```python
from build123d import *

# Parameters (mm, degrees)
SKETCH1_R           = 4.25
BOSS_EXTRUDE1_DEPTH = 55.3238373
CUT_EXTRUDE1_DEPTH  = 6.6
CHAMFER1_SIZE       = 0.5
CUT_EXTRUDE2_DEPTH  = 6.6
CHAMFER2_SIZE       = 0.5


with BuildPart() as part:
    # Sketch1 → Boss-Extrude1 (new body)
    with BuildSketch(Plane(origin=(0, 0, 0), x_dir=(1, 0, 0), z_dir=(0, 1, 0))):
        Circle(SKETCH1_R)
    extrude(amount=BOSS_EXTRUDE1_DEPTH)

    # Sketch2 → Cut-Extrude1 (cut)
    with BuildSketch(Plane(origin=(0, 55.3238373, 0), x_dir=(1, 0, 0), z_dir=(0, 1, 0))):
        Polygon((1.610807251, 2.79), (-1.610807251, 2.79), (-3.221614502, 0), (-1.610807251, -2.79), (1.610807251, -2.79), (3.221614502, 0), align=None)
    extrude(amount=-CUT_EXTRUDE1_DEPTH, mode=Mode.SUBTRACT)

    # Chamfer1
    chamfer1_edges = [part.edges().sort_by_distance(p)[0] for p in [
        (2.416210877, 55.3238373, -1.395),
        (0, 55.3238373, -2.79),
        (-2.416210877, 55.3238373, -1.395),
        (-2.416210877, 55.3238373, 1.395),
        (0, 55.3238373, 2.79),
        (2.416210877, 55.3238373, 1.395),
    ]]
    chamfer(chamfer1_edges, length=CHAMFER1_SIZE)

    # Sketch3 → Cut-Extrude2 (cut)
    with BuildSketch(Plane.XZ):
        Polygon((0, 3.221614502), (-2.79, 1.610807251), (-2.79, -1.610807251), (0, -3.221614502), (2.79, -1.610807251), (2.79, 1.610807251), align=None)
    extrude(amount=-CUT_EXTRUDE2_DEPTH, mode=Mode.SUBTRACT)

    # Chamfer2
    chamfer2_edges = [part.edges().sort_by_distance(p)[0] for p in [
        (1.395, 0, 2.416210877),
        (-1.395, 0, 2.416210877),
        (-2.79, 0, 0),
        (-1.395, 0, -2.416210877),
        (1.395, 0, -2.416210877),
        (2.79, 0, 0),
    ]]
    chamfer(chamfer2_edges, length=CHAMFER2_SIZE)


solid = part.part
```
Read the model definition and answer for the solid it produces. Units are mm, in the model's axes. A direction names the side the tool comes from. Give positions to 0.01 mm unless a question says otherwise; leave off trailing zeros. Write each loop counter-clockwise with the first axis right and the second up, starting at its lowest first coordinate (ties: lowest second). Pieces come first, ordered by that corner, then holes. Notation, with made-up numbers: (52, 35.25) -> (68, 35.25) arc R23 ccw to (68, 56.25) -> close; hole circle Ø3 at (-8.5, 24). An arc over 180 degrees is marked (long way). Answer as a JSON object with one key per item and string values.
1) A tool of negligible diameter and unlimited length cuts with its end or side. For faces 3 (the flat face through (-2.64, 55.07, 1.5)), 4 (the flat face through (2.79, 4, 0)), from which of +Z, -Z, +X, -X, +Y, -Y can it reach the whole face along a straight path? Write none if from no direction.
Findings below:
{"face 3": "+Y", "face 4": "-Y"}
2) For a pull along Z with two mould halves and no side action, classify faces 1 (the cylindrical face through (2.285, 27.275, -3.584)), 2 (the flat face through (2.405, 51.817, 1.415)) as pulls with the +Z half, pulls with the -Z half, needs draft (parallel to the pull), parting line crosses it, or undercut.
Findings below:
{"face 1": "parting line crosses it", "face 2": "undercut"}
3) Section B-B on x = 0.5 is taken. Write down the section's boundary in (y, z).
Findings below:
{"outline": "(0, -4.22) -> (55.32, -4.22) -> (55.32, -3.29) -> (54.82, -2.79) -> (48.72, -2.79) -> (48.72, 2.79) -> (54.82, 2.79) -> (55.32, 3.29) -> (55.32, 4.22) -> (0, 4.22) -> (0, 3.51) -> (0.5, 2.93) -> (6.6, 2.93) -> (6.6, -2.93) -> (0.5, -2.93) -> (0, -3.51) -> close"}
4) Flat-ended cylindrical pins translate along their axes: pin 1 Ø3 at (x, z) = (1.5, 0.5) entering from -Y; pin 2 Ø2 at (y, z) = (7, 1.5) entering from -X; pin 3 Ø2 at (x, y) = (3, 17) entering from +Z. Find the tip coordinate at first contact, or state that the pin passes through.
Findings below:
{"pin 1": "stops at y = 0.29", "pin 2": "stops at x = -4.22", "pin 3": "stops at z = 3.75"}
5) Straight lines are drawn through the part: probe 1 along X at (y, z) = (3, 0); probe 2 along Z at (x, y) = (0.25, 16); probe 3 along Z at (x, y) = (-1.25, 51). For each, find the intervals that lie inside material, in ascending order. Write a range as from..to.
Findings below:
{"probe 1": "x = -4.25..-2.79, 2.79..4.25", "probe 2": "z = -4.24..4.24", "probe 3": "z = -4.06..-2.79, 2.79..4.06"}
6) Section C-C on y = 10.5 is taken. Write down the section's boundary in (x, z), then the cut area to 3 significant figures.
Findings below:
{"outline": "circle Ø8.5 at (0, 0)", "area": "56.7 mm^2"}
7) Section A-A on y = 50.5 is taken. Write down the section's boundary in (x, z), then the cut area to 3 significant figures.
Findings below:
{"outline": "circle Ø8.5 at (0, 0); hole (-3.22, 0) -> (-1.61, -2.79) -> (1.61, -2.79) -> (3.22, 0) -> (1.61, 2.79) -> (-1.61, 2.79) -> close", "area": "29.8 mm^2"}
